Job drawing, mm, ordinate dimensions from the low corner. One solid piece. A direction names the side the tool comes from. Round coordinates to 2 decimals unless told otherwise and drop trailing zeros. Write each loop counter-clockwise with the first axis right and the second up, starting at its lowest first coordinate (ties: lowest second). Pieces come first, ordered by that corner, then holes.
1) Saw through at B-B (x = 39). Write the cut outline in (y, z) (1 decimal).
2) Saw through at C-C (y = 16.5). Write the cut outline in (x, z) (1 decimal).
3) Wall check: probe 1 along X at (y, z) = (5.5, 0.25); probe 2 along Y at (x, z) = (42.5, 1.4); probe 3 along X at (y, z) = (10, 4.55) (1 decimal). Give the ranges that are in metal, low to high.
4) Which spindle directions (+Z, -Z, +X, -X, +Y, -Y) get a long thin tool onto all of the face, cutting with end or side? Do the marked faces 1 and 2. Say none if no direction does.
5) Saw through at D-D (z = 4.15). State how many separate pieces and enclosed holes the cut face has, plus the area to 3 significant figures.
6) Saw through at A-A (z = 0.6). Write the cut outline in (x, y).
7) Flat gauge pins, fed straight in: pin 1 (1.2 mm diameter, centred on x = 27.81, y = 19.89, fed in from -Z) (1 decimal); pin 2 (0.5 mm diameter, centred on x = 4, y = 28, fed in from -Z) (3 decimals). Where does each tip first touch, or does it go through?
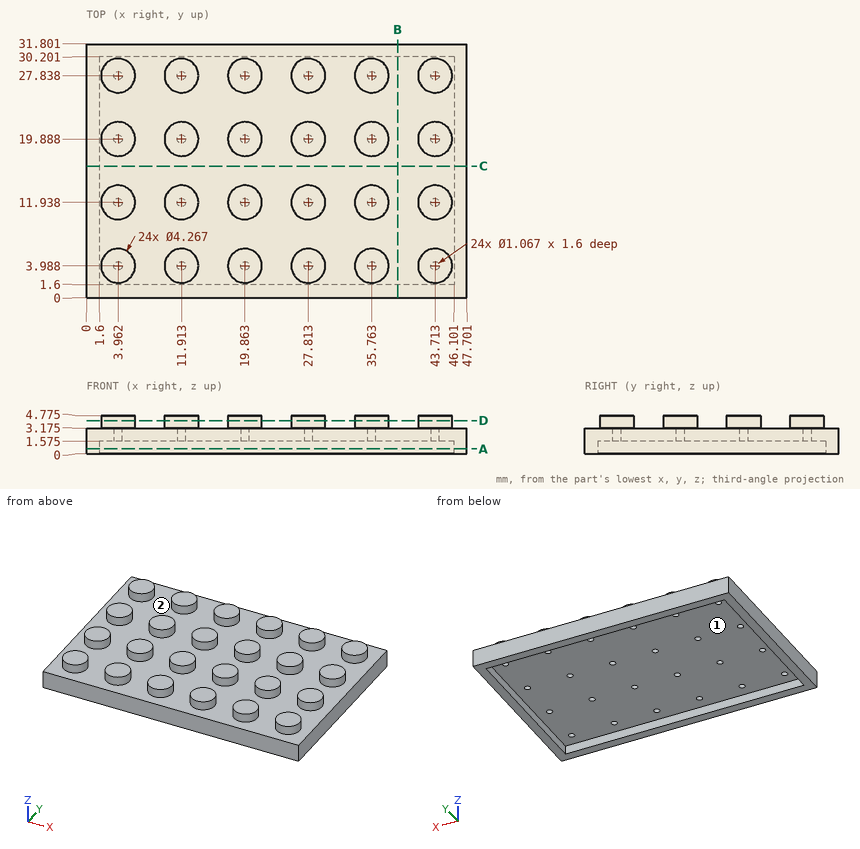
Evaluation:
1. outline: (0, 0) - (1.6, 0) - (1.6, 1.6) - (30.2, 1.6) - (30.2, 0) - (31.8, 0) - (31.8, 3.2) - (0, 3.2) - close
2. outline: (0, 0) - (1.6, 0) - (1.6, 1.6) - (46.1, 1.6) - (46.1, 0) - (47.7, 0) - (47.7, 3.2) - (0, 3.2) - close
3. probe 1: x = 0 to 1.6, 46.1 to 47.7
3. probe 2: y = 0 to 1.6, 30.2 to 31.8
3. probe 3: x = 3.1 to 4.9, 11 to 12.8, 19 to 20.8, 26.9 to 28.7, 34.9 to 36.7, 42.8 to 44.6
4. face 1: -Z
4. face 2: +Z
5. separate pieces: 24
5. enclosed holes: 0
5. area: 343 mm2
6. outline: (0, 0) - (47.7, 0) - (47.7, 31.8) - (0, 31.8) - close; hole (1.6, 1.6) - (46.1, 1.6) - (46.1, 30.2) - (1.6, 30.2) - close
7. pin 1: stops at z = 1.6
7. pin 2: stops at z = 3.175
